Can you work these out from the model? Positions are in its coordinate system, mm. A direction names the side the tool comes from. Give positions to 0.01 mm unless a question says otherwise; leave off trailing zeros. Loops run counter-clockwise (first coordinate to the right, second up) from the corner with the lowest first, then second, coordinate; pieces in that order, holes last. Notation, with made-up numbers: (47.25, -15.75) - (73.25, -15.75) arc R22 cw to (73.25, 12.25) - close; hole circle Ø8 at (-39.75, 76.5). An arc over 180 degrees is marked (long way). Answer as a JSON object with one key per item and string values. Group by question number.
Item 1: Suppose I cut it at B-B on x = 7. Write out the boundary of the cut face in (y, z) (3 decimals), and give its area (3 significant figures).
Item 2: Suppose I cut it at D-D on y = -5. Write out the boundary of the cut face in (x, z) (3 decimals).
Item 3: Will these pins go through, and if not, where does the flat tip stop? pin 1 (3 mm diameter, centred on y = 5, z = -3.5, fed in from +X); pin 2 (4 mm diameter, centred on y = -5, z = -3.5, fed in from +X).
Item 4: Suppose I cut it at A-A on y = 5. Write out the boundary of the cut face in (x, z) (3 decimals), and give its area (3 significant figures).
Item 5: Which directions (+Z, -Z, +X, -X, +Y, -Y) give clear straight access to the entire face, cutting with the end or side of a thin tool? Please do faces 1 (the flat face through (0, 0, 0)), 2 (the cylindrical face through (1.964, -6.474, -3.435)).
Item 6: Suppose I cut it at C-C on z = -3.5. Write out the boundary of the cut face in (x, y) (3 decimals), and give its area (3 significant figures).
Item 7: Please list where these lines run through material, in increasing order: L1, parallel to Z at x = 2.75, y = 5 (3 decimals); L2, parallel to Y at x = 1.5, z = -3; L3, parallel to Y at x = 1.75, z = -3.25.
from build123d import *

# Parameters (mm, degrees)
F0_W         = 20
F0_H         = 16
F1_DEPTH     = 7
F2_R         = 0.5
F3_T1_DEPTH  = 22.5
F3_T3_DEPTH  = 16.75
F3_T5_DEPTH  = 6
F3_S9_W      = 0.5
F3_S9_H      = 0.5
F3_T10_DEPTH = 0.5
F3_S15_W     = 0.5
F3_S15_H     = 0.5
F3_T16_DEPTH = 0.5
F3_T20_ANGLE = 90
F3_T22_ANGLE = 90
F4_T1_DEPTH  = 6
F4_S5_W      = 0.5
F4_S5_H      = 0.5
F4_T6_DEPTH  = 0.5
F4_S11_W     = 0.5
F4_S11_H     = 0.5
F4_T12_DEPTH = 0.5
F5_T1_DEPTH  = 6
F5_S5_W      = 0.5
F5_S5_H      = 0.5
F5_T6_DEPTH  = 0.5
F5_S11_W     = 0.5
F5_S11_H     = 0.5
F5_T12_DEPTH = 0.5
F6_R         = 1.475
F6_R_2       = 1.725
F7_DEPTH     = 16.3


# Not quite as in the source:
# - a fillet or chamfer that OpenCascade refuses, or shapes differently, is made with other operations: its cross-section is extruded or revolved along the edge and cut away or added


with BuildPart() as f1:
    # F0 (on Top) → F1 (new body)
    with BuildSketch(Plane.XY):
        Rectangle(F0_W, F0_H)
    extrude(amount=-F1_DEPTH)

    # F2
    f2_edges = [f1.edges().sort_by_distance(p)[0] for p in [
        (0, 8, 0),
        (-10, 0, 0),
        (0, -8, 0),
        (10, 0, 0),
        (0, -8, -7),
    ]]
    fillet(f2_edges, radius=F2_R)

    # F3: fillet of radius 0.5 on 4 edges, made by hand

    # F3_s2 → F3_t1 (cut)
    with BuildSketch(Plane.YZ.offset(-11.25)):
        with BuildLine():
            ThreePointArc((8, -6.5), (7.8535533906, -6.8535533906), (7.5, -7))
            Line((7.5, -7), (8, -7))
            Line((8, -7), (8, -6.5))
        make_face()
    extrude(amount=F3_T1_DEPTH, mode=Mode.SUBTRACT)

    # F3_s4 → F3_t3 (cut)
    with BuildSketch(Plane.XZ.offset(-9.25)):
        with BuildLine():
            ThreePointArc((-9.5, -7), (-9.8535533906, -6.8535533906), (-10, -6.5))
            Line((-10, -6.5), (-10, -7))
            Line((-10, -7), (-9.5, -7))
        make_face()
        with BuildLine():
            ThreePointArc((10, -6.5), (9.8535533906, -6.8535533906), (9.5, -7))
            Line((9.5, -7), (10, -7))
            Line((10, -7), (10, -6.5))
        make_face()
    extrude(amount=F3_T3_DEPTH, mode=Mode.SUBTRACT)

    # F3_s6 → F3_t5 (cut)
    with BuildSketch(Plane.XY.offset(-6.5)):
        with BuildLine():
            ThreePointArc((10, -7.5), (9.8535533906, -7.8535533906), (9.5, -8))
            Line((9.5, -8), (10, -8))
            Line((10, -8), (10, -7.5))
        make_face()
        with BuildLine():
            ThreePointArc((-10, -7.5), (-9.8535533906, -7.8535533906), (-9.5, -8))
            Line((-9.5, -8), (-10, -8))
            Line((-10, -8), (-10, -7.5))
        make_face()
    extrude(amount=F3_T5_DEPTH, mode=Mode.SUBTRACT)


with BuildPart() as f3_tool8:
    # F3_s9 → F3_t10 (new body)
    with BuildSketch(Plane.YZ.offset(9.5)):
        with Locations((-7.75, -0.25)):
            Rectangle(F3_S9_W, F3_S9_H)
    extrude(amount=F3_T10_DEPTH)

    # F3_s11 → F3_t12 (revolve, cut)
    with BuildSketch(Plane(origin=(9.5, -7.5, -0.5), x_dir=(0, 0.7071067812, -0.7071067812), z_dir=(0, -0.7071067812, -0.7071067812))):
        with BuildLine():
            ThreePointArc((0, -0.5), (0.5, 0), (0, 0.5))
            Line((0, 0.5), (0, -0.5))
        make_face()
    revolve(axis=Axis((9.5, -7.5, -0.5), (1, 0, 0)), mode=Mode.SUBTRACT)


with BuildPart() as f1_1:
    add(f1.part)

    # F3_t7: cut F3_tool8
    add(f3_tool8.part, mode=Mode.SUBTRACT)


with BuildPart() as f3_tool14:
    # F3_s15 → F3_t16 (new body)
    with BuildSketch(Plane.YZ.offset(-9.5)):
        with Locations((-7.75, -0.25)):
            Rectangle(F3_S15_W, F3_S15_H)
    extrude(amount=-F3_T16_DEPTH)

    # F3_s17 → F3_t18 (revolve, cut)
    with BuildSketch(Plane(origin=(-9.5, -7.5, -0.5), x_dir=(0, 0.7071067812, -0.7071067812), z_dir=(0, 0.7071067812, 0.7071067812))):
        with BuildLine():
            ThreePointArc((0, -0.5), (0.5, 0), (0, 0.5))
            Line((0, 0.5), (0, -0.5))
        make_face()
    revolve(axis=Axis((-9.5, -7.5, -0.5), (-1, 0, 0)), mode=Mode.SUBTRACT)


with BuildPart() as f1_2:
    add(f1_1.part)

    # F3_t13: cut F3_tool14
    add(f3_tool14.part, mode=Mode.SUBTRACT)

    # F3_s19 → F3_t20 (revolve, cut)
    with BuildSketch(Plane.XY.offset(-6.5)):
        with BuildLine():
            ThreePointArc((10, -7.5), (9.8535533906, -7.8535533906), (9.5, -8))
            Line((9.5, -8), (10, -8))
            Line((10, -8), (10, -7.5))
        make_face()
    revolve(axis=Axis((10, -7.5, -6.5), (1, 0, 0)), revolution_arc=F3_T20_ANGLE, mode=Mode.SUBTRACT)

    # F3_s21 → F3_t22 (revolve, cut)
    with BuildSketch(Plane.XY.offset(-6.5)):
        with BuildLine():
            ThreePointArc((-10, -7.5), (-9.8535533906, -7.8535533906), (-9.5, -8))
            Line((-9.5, -8), (-10, -8))
            Line((-10, -8), (-10, -7.5))
        make_face()
    revolve(axis=Axis((-10, -7.5, -6.5), (1, 0, 0)), revolution_arc=F3_T22_ANGLE, mode=Mode.SUBTRACT)

    # F4: fillet of radius 0.5 on 1 edges, made by hand

    # F4_s2 → F4_t1 (cut)
    with BuildSketch(Plane.XY.offset(-6.5)):
        with BuildLine():
            ThreePointArc((-9.5, 8), (-9.8535533906, 7.8535533906), (-10, 7.5))
            Line((-10, 7.5), (-10, 8))
            Line((-10, 8), (-9.5, 8))
        make_face()
    extrude(amount=F4_T1_DEPTH, mode=Mode.SUBTRACT)


with BuildPart() as f4_tool4:
    # F4_s5 → F4_t6 (new body)
    with BuildSketch(Plane.XZ.offset(-7.5)):
        with Locations((-9.75, -0.25)):
            Rectangle(F4_S5_W, F4_S5_H)
    extrude(amount=-F4_T6_DEPTH)

    # F4_s7 → F4_t8 (revolve, cut)
    with BuildSketch(Plane(origin=(-9.5, 7.5, -0.5), x_dir=(0.7071067812, 0, -0.7071067812), z_dir=(0.7071067812, 0, 0.7071067812))):
        with BuildLine():
            ThreePointArc((0, -0.5), (0.5, 0), (0, 0.5))
            Line((0, 0.5), (0, -0.5))
        make_face()
    revolve(axis=Axis((-9.5, 7.5, -0.5), (0, 1, 0)), mode=Mode.SUBTRACT)


with BuildPart() as f1_3:
    add(f1_2.part)

    # F4_t3: cut F4_tool4
    add(f4_tool4.part, mode=Mode.SUBTRACT)


with BuildPart() as f4_tool10:
    # F4_s11 → F4_t12 (new body)
    with BuildSketch(Plane.XZ.offset(-7.5)):
        with Locations((-9.75, -6.75)):
            Rectangle(F4_S11_W, F4_S11_H)
    extrude(amount=-F4_T12_DEPTH)

    # F4_s13 → F4_t14 (revolve, cut)
    with BuildSketch(Plane(origin=(-9.5, 7.5, -6.5), x_dir=(0.7071067812, 0, 0.7071067812), z_dir=(-0.7071067812, 0, 0.7071067812))):
        with BuildLine():
            ThreePointArc((0, -0.5), (0.5, 0), (0, 0.5))
            Line((0, 0.5), (0, -0.5))
        make_face()
    revolve(axis=Axis((-9.5, 7.5, -6.5), (0, 1, 0)), mode=Mode.SUBTRACT)


with BuildPart() as f1_4:
    add(f1_3.part)

    # F4_t9: cut F4_tool10
    add(f4_tool10.part, mode=Mode.SUBTRACT)

    # F5: fillet of radius 0.5 on 1 edges, made by hand

    # F5_s2 → F5_t1 (cut)
    with BuildSketch(Plane.XY.offset(-6.5)):
        with BuildLine():
            ThreePointArc((9.5, 8), (9.8535533906, 7.8535533906), (10, 7.5))
            Line((10, 7.5), (10, 8))
            Line((10, 8), (9.5, 8))
        make_face()
    extrude(amount=F5_T1_DEPTH, mode=Mode.SUBTRACT)


with BuildPart() as f5_tool4:
    # F5_s5 → F5_t6 (new body)
    with BuildSketch(Plane.XZ.offset(-7.5)):
        with Locations((9.75, -0.25)):
            Rectangle(F5_S5_W, F5_S5_H)
    extrude(amount=-F5_T6_DEPTH)

    # F5_s7 → F5_t8 (revolve, cut)
    with BuildSketch(Plane(origin=(9.5, 7.5, -0.5), x_dir=(-0.7071067812, 0, -0.7071067812), z_dir=(0.7071067812, 0, -0.7071067812))):
        with BuildLine():
            ThreePointArc((0, -0.5), (0.5, 0), (0, 0.5))
            Line((0, 0.5), (0, -0.5))
        make_face()
    revolve(axis=Axis((9.5, 7.5, -0.5), (0, 1, 0)), mode=Mode.SUBTRACT)


with BuildPart() as f1_5:
    add(f1_4.part)

    # F5_t3: cut F5_tool4
    add(f5_tool4.part, mode=Mode.SUBTRACT)


with BuildPart() as f5_tool10:
    # F5_s11 → F5_t12 (new body)
    with BuildSketch(Plane.XZ.offset(-7.5)):
        with Locations((9.75, -6.75)):
            Rectangle(F5_S11_W, F5_S11_H)
    extrude(amount=-F5_T12_DEPTH)

    # F5_s13 → F5_t14 (revolve, cut)
    with BuildSketch(Plane(origin=(9.5, 7.5, -6.5), x_dir=(-0.7071067812, 0, 0.7071067812), z_dir=(-0.7071067812, 0, -0.7071067812))):
        with BuildLine():
            ThreePointArc((0, -0.5), (0.5, 0), (0, 0.5))
            Line((0, 0.5), (0, -0.5))
        make_face()
    revolve(axis=Axis((9.5, 7.5, -6.5), (0, 1, 0)), mode=Mode.SUBTRACT)


with BuildPart() as f1_6:
    add(f1_5.part)

    # F5_t9: cut F5_tool10
    add(f5_tool10.part, mode=Mode.SUBTRACT)

    # F6 (on face) → F7 (cut)
    with BuildSketch(Plane.YZ.offset(10)):
        with Locations((-5, -3.5)):
            Circle(F6_R)
        with Locations((5, -3.5)):
            Circle(F6_R_2)
    extrude(amount=-F7_DEPTH, mode=Mode.SUBTRACT)


solid = f1_6.part
Worked out:
{
 "1": {"outline": "(-8, -6.5) arc R0.5 ccw to (-7.5, -7) - (7.5, -7) arc R0.5 ccw to (8, -6.5) - (8, -0.5) arc R0.5 ccw to (7.5, 0) - (-7.5, 0) arc R0.5 ccw to (-8, -0.5) - close; hole circle Ø2.95 at (-5, -3.5); hole circle Ø3.45 at (5, -3.5)", "area": "95.6 mm2"},
 "2": {"outline": "(-10, -6.5) arc R0.5 ccw to (-9.5, -7) - (9.5, -7) arc R0.5 ccw to (10, -6.5) - (10, -4.975) - (-6.3, -4.975) - (-6.3, -2.025) - (10, -2.025) - (10, -0.5) arc R0.5 ccw to (9.5, 0) - (-9.5, 0) arc R0.5 ccw to (-10, -0.5) - close"},
 "3": {"pin 1": "stops at x = -6.3", "pin 2": "stops at x = 10"},
 "4": {"outline": "(-10, -6.5) arc R0.5 ccw to (-9.5, -7) - (9.5, -7) arc R0.5 ccw to (10, -6.5) - (10, -5.225) - (-6.3, -5.225) - (-6.3, -1.775) - (10, -1.775) - (10, -0.5) arc R0.5 ccw to (9.5, 0) - (-9.5, 0) arc R0.5 ccw to (-10, -0.5) - close", "area": "83.6 mm2"},
 "5": {"face 1": "+Z, +X, -X, +Y, -Y", "face 2": "+X"},
 "6": {"outline": "(-10, -7.5) arc R0.5 ccw to (-9.5, -8) - (9.5, -8) arc R0.5 ccw to (10, -7.5) - (10, -6.475) - (-6.3, -6.475) - (-6.3, -3.525) - (10, -3.525) - (10, 3.275) - (-6.3, 3.275) - (-6.3, 6.725) - (10, 6.725) - (10, 7.5) arc R0.5 ccw to (9.5, 8) - (-9.5, 8) arc R0.5 ccw to (-10, 7.5) - close", "area": "215 mm2"},
 "7": {"L1": "z = -7 to -5.225, -1.775 to 0", "L2": "y = -8 to -6.39, -3.61 to 3.35, 6.65 to 8", "L3": "y = -8 to -6.45, -3.55 to 3.29, 6.71 to 8"}
}
